```python
from build123d import *

# Parameters (mm, degrees)
F0_W     = 83.82
F0_H     = 154.94
F1_DEPTH = 12.7
F2_W     = 71.12
F2_H     = 142.24
F3_DEPTH = 7.62
F4_R     = 5.08
F5_R     = 5.08
F6_R     = 5.08
F7_R     = 5.08


with BuildPart() as f1:
    # F0 (on Top) → F1 (new body)
    with BuildSketch(Plane.XY):
        Rectangle(F0_W, F0_H)
    extrude(amount=F1_DEPTH)

    # F2 (on Top) → F3 (cut)
    with BuildSketch(Plane.XY):
        Rectangle(F2_W, F2_H)
    extrude(amount=F3_DEPTH, mode=Mode.SUBTRACT)

    # F4
    f4_edges = [f1.edges().sort_by_distance(p)[0] for p in [
        (41.91, -77.47, 6.35),
    ]]
    fillet(f4_edges, radius=F4_R)

    # F5
    f5_edges = [f1.edges().sort_by_distance(p)[0] for p in [
        (41.91, 77.47, 6.35),
    ]]
    fillet(f5_edges, radius=F5_R)

    # F6
    f6_edges = [f1.edges().sort_by_distance(p)[0] for p in [
        (-41.91, -77.47, 6.35),
    ]]
    fillet(f6_edges, radius=F6_R)

    # F7
    f7_edges = [f1.edges().sort_by_distance(p)[0] for p in [
        (-41.91, 77.47, 6.35),
    ]]
    fillet(f7_edges, radius=F7_R)

    # F10: sweep along a path in F9
    with BuildLine(Plane.YZ) as f10_path:
        Line((-68.238609, 13.756951), (-109.795533, 111.935183))
    # F8 (on face) → F10 (sweep)
    with BuildSketch(Plane.XY.offset(12.7)):
        with BuildLine():
            ThreePointArc((12.210004, -77.47), (14.725381, -73.015905), (15.59766, -67.975546))
            ThreePointArc((15.59766, -67.975546), (-4.441399, -53.849124), (-11.012084, -77.47))
            Line((-11.012084, -77.47), (12.210004, -77.47))
        make_face()
    sweep(path=f10_path.line)

    # F11: F1 across plane


with BuildPart() as f1_1:
    add(f1.part)
    add(f1.part.mirror(Plane.XZ))


solid = f1_1.part
```
CAD build for the part. Positions are in the model's coordinates, mm. A direction names the side the tool comes from. Round coordinates to 2 decimals unless told otherwise and drop trailing zeros. Order: outer loops, then holes, each group sorted by start corner. A loop starts at its lowest first (then second) coordinate and runs counter-clockwise, first axis right, second up.
Q1. Wall check: L1, parallel to Z at x = -1, y = 46; L2, parallel to X at y = -2.5, z = 6.5; L3, parallel to Y at x = 1.5, z = 23. Give the ranges that are in metal, low to high.
Q2. Two-plate mould, pull along Y, no slides. Class faces 4 (the flat face through (-35.56, -1, 4)), 5 (the flat face through (-1, 77.47, 6)), 6 (the flat face through (-37, 6, 0)): pulls with the +Y half, pulls with the -Y half, needs draft (parallel to the pull), parting line crosses it, or undercut.
Q3. Drop flat-ended pins along their axis: pin 1 (4 mm diameter, centred on x = -10, y = -20, fed in from +Z); pin 2 (4 mm diameter, centred on x = 13.5, z = 16, fed in from -Y); pin 3 (3 mm diameter, centred on y = -70, z = 37.5, fed in from +X); pin 4 (8 mm diameter, centred on x = 20, z = 21, fed in from -Y). Give the stop position or say it passes through.
Q4. Which spindle directions (+Z, -Z, +X, -X, +Y, -Y) get a long thin tool onto all of the face, cutting with end or side? Do faces 1 (the flat face through (0, 71.12, 4)), 2 (the flat face through (-1, -77.47, 6)), 3 (the flat face through (0, -107, 110.878)). Say none if no direction does.
Q5. Slice it at B-B (y = -39.5). Write the cut outline in (x, z), and give its area (3 significant figures).
Q6. Slice it at A-A (x = 20.5). Write the cut outline in (y, z), and give its area (3 significant figures).
Results below:
1. L1: z = 7.62 to 12.7
1. L2: x = -41.91 to -35.56, 35.56 to 41.91
1. L3: y = -81.83 to -57.36, 57.36 to 81.83
2. face 4: undercut
2. face 5: pulls with the +Y half
2. face 6: needs draft
3. pin 1: stops at z = 12.7
3. pin 2: stops at y = -79.51
3. pin 3: stops at x = 13.95
3. pin 4: passes through
4. face 1: -Z
4. face 2: -Z, +X, -X, -Y
4. face 3: +Z, +X, -X, +Y, -Y
5. outline: (-41.91, 0) - (-35.56, 0) - (-35.56, 7.62) - (35.56, 7.62) - (35.56, 0) - (41.91, 0) - (41.91, 12.7) - (-41.91, 12.7) - close
5. area: 523 mm2
6. outline: (-77.47, 0) - (-71.12, 0) - (-71.12, 7.62) - (71.12, 7.62) - (71.12, 0) - (77.47, 0) - (77.47, 12.7) - (-77.47, 12.7) - close
6. area: 884 mm2
